```python
from build123d import *

# Parameters (mm, degrees)
SKETCH_1_R          = 15
EXTRUDE_1_DEPTH     = 5.5
SKETCH_2_R          = 6
EXTRUDE_2_DEPTH     = 2
SKETCH_3_R          = 5
EXTRUDE_3_DEPTH     = 7.5
SKETCH_4_R          = 1.65
CUT_EXTRUDE_1_DEPTH = 26.980762114


with BuildPart() as part:
    # ｽｹｯﾁ1 → ﾎﾞｽ - 押し出し1 (new body)
    with BuildSketch(Plane(origin=(0, 0, 0), x_dir=(0, 0, -1), z_dir=(1, 0, 0))):
        Circle(SKETCH_1_R)
    extrude(amount=EXTRUDE_1_DEPTH)

    # ｽｹｯﾁ2 → ﾎﾞｽ - 押し出し2 (add)
    with BuildSketch(Plane.ZY):
        Circle(SKETCH_2_R)
    extrude(amount=EXTRUDE_2_DEPTH)

    # ｽｹｯﾁ3 → ﾎﾞｽ - 押し出し3 (add)
    with BuildSketch(Plane.ZY.offset(2)):
        Circle(SKETCH_3_R)
    extrude(amount=EXTRUDE_3_DEPTH)

    # ｽｹｯﾁ4 → ｶｯﾄ - 押し出し1 (cut, through all)
    with BuildSketch(Plane(origin=(5.5, 0, 0), x_dir=(0, 0, -1), z_dir=(1, 0, 0))):
        with Locations((10, 0)):
            Circle(SKETCH_4_R)
        with Locations((-10, 0)):
            Circle(SKETCH_4_R)
    extrude(amount=-CUT_EXTRUDE_1_DEPTH, mode=Mode.SUBTRACT)


solid = part.part
```
Could you check a few things on this model? Use its own coordinates, in mm. A direction names the side the tool comes from. Round coordinates to 2 decimals unless told otherwise and drop trailing zeros. Loops run counter-clockwise (first coordinate to the right, second up) from the corner with the lowest first, then second, coordinate; pieces in that order, holes last. Notation, with made-up numbers: (32, -9.75) -> (81, -9.75) arc R13 ccw to (81, 7.25) -> close; hole circle Ø3 at (51, 43.5). An arc over 180 degrees is marked (long way). Put each result on its own line as item: value.
Q1. Which directions (+Z, -Z, +X, -X, +Y, -Y) give clear straight access to the entire face, cutting with the end or side of a thin tool? Please do faces 4 (the cylindrical face through (-1, 0, -6)), 5 (the flat face through (5.5, 0, 0)).
Checks:
face 4: -X
face 5: +Z, -Z, +X, +Y, -Y
Q2. Thinking about a two-plate mould opening in Y: for faces 1 (the cylindrical face through (-5.7, -4.88, -1.08)), 2 (the flat face through (-9.5, 0, 0)), 3 (the cylindrical face through (2.788, -0.632, 8.476)), which applies, pulls with the +Y half, pulls with the -Y half, needs draft (parallel to the pull), parting line crosses it, or undercut?
Checks:
face 1: parting line crosses it
face 2: needs draft
face 3: undercut
Q3. I want a section at C-C on z = 10. Write out the boundary of the cut face in (x, y), and give its area (3 significant figures).
Checks:
outline: (0, -11.18) -> (5.5, -11.18) -> (5.5, -1.65) -> (0, -1.65) -> close; (0, 1.65) -> (5.5, 1.65) -> (5.5, 11.18) -> (0, 11.18) -> close
area: 105 mm2
Q4. I want a section at B-B on z = 0. Write out the boundary of the cut face in (x, y), and give its area (3 significant figures).
Checks:
outline: (-9.5, -5) -> (-2, -5) -> (-2, -6) -> (0, -6) -> (0, -15) -> (5.5, -15) -> (5.5, 15) -> (0, 15) -> (0, 6) -> (-2, 6) -> (-2, 5) -> (-9.5, 5) -> close
area: 264 mm2
Q5. I want a section at D-D on y = -3. Write out the boundary of the cut face in (x, z), and give its area (3 significant figures).
Checks:
outline: (-9.5, -4) -> (-2, -4) -> (-2, -5.2) -> (0, -5.2) -> (0, -14.7) -> (5.5, -14.7) -> (5.5, 14.7) -> (0, 14.7) -> (0, 5.2) -> (-2, 5.2) -> (-2, 4) -> (-9.5, 4) -> close
area: 242 mm2
Q6. Please list where these lines run through material, in increasing order: line 1 (X direction, y = 5.25, z = -0.75); line 2 (X direction, y = 7.5, z = -4); line 3 (Y direction, x = 3.9, z = 10). Write a range as from..to.
Checks:
line 1: -2..5.5
line 2: 0..5.5
line 3: -11.18..-1.65, 1.65..11.18
Q7. I want a section at A-A on y = 0. Write out the boundary of the cut face in (x, z).
Checks:
outline: (-9.5, -5) -> (-2, -5) -> (-2, -6) -> (0, -6) -> (0, -8.35) -> (5.5, -8.35) -> (5.5, 8.35) -> (0, 8.35) -> (0, 6) -> (-2, 6) -> (-2, 5) -> (-9.5, 5) -> close; (0, -15) -> (5.5, -15) -> (5.5, -11.65) -> (0, -11.65) -> close; (0, 11.65) -> (5.5, 11.65) -> (5.5, 15) -> (0, 15) -> close
Q8. For pin 1 Ø4 at (y, z) = (-8, 10) entering from -X; pin 2 Ø5 at (x, z) = (0.5, -5) entering from +Y; pin 3 Ø1 at (x, z) = (-6.5, -2.5) entering from +Y, each with a flat end and sliding along its axis, tell me the tip position at first contact or that it passes through.
Checks:
pin 1: x = 0
pin 2: y = 14.79
pin 3: y = 4.58
